The listing builds one solid part. Answer for the finished solid, in the listing's coordinates (mm). A direction names the side the tool comes from. Round coordinates to 2 decimals unless told otherwise and drop trailing zeros. Order: outer loops, then holes, each group sorted by start corner. A loop starts at its lowest first (then second) coordinate and runs counter-clockwise, first axis right, second up. Notation, with made-up numbers: (-9, 62.5) - (34, 62.5) arc R28 cw to (34, 96.5) - close; hole circle Ø7 at (11, 68.5). An arc over 180 degrees is marked (long way). One line per item, written item: value. Start each with the question number.
1. Section A-A, the plane x = 0 is taken. Give the vertices of the cut face in (y, z).
2. A tool of negligible diameter and unlimited length cuts with its end or side. For faces 1 (the flat face through (5.5, -3.12, 3.94)), 2 (the cylindrical face through (2.38, 10.74, 59.04)), 3 (the flat face through (10, -10, 64)), from which of +Z, -Z, +X, -X, +Y, -Y can it reach the whole face along a straight path? Write none if from no direction.
3. Flat-ended cylindrical pins translate along their axes: P1, Ø13, axis at x = 0, y = 0, coming from the +Z side; P2, Ø1.5, axis at y = 12.5, z = 20.5, coming from the +X side; P3, Ø10, axis at x = 15.5, z = 45.5, coming from the +Y side; P4, Ø14, axis at x = 2.5, y = 2.5, coming from the -Z side. Find the tip coordinate at first contact, or state that the pin passes through.
4. Straight lines are drawn through the part: line 1 (Z direction, x = 6, y = 6.5); line 2 (Y direction, x = 0, z = 24); line 3 (Y direction, x = 0, z = 57). For each, find the intervals that lie inside material, in ascending order.
5. For a pull along Y with two mould halves and no side action, classify faces 4 (the flat face through (0, -6.322, 4)), 5 (the flat face through (3, -3, 8)), 6 (the flat face through (0, -8, 0)), 7 (the conical face through (22.72, 7.15, 33.76)) as released by +Y, released by -Y, zero draft, split by the parting line, or undercut.
6. Section B-B, the plane z = 37 is taken. Give the vertices of the cut face in (x, y).
from build123d import *

# Parameters (mm, degrees)
POCKET_DEPTH    = 8
SKETCH003_R     = 3.95
POCKET001_DEPTH = 64.001
SKETCH004_R     = 11
POCKET002_DEPTH = 8
FILLET_R        = 2
FILLET001_R     = 5


with BuildPart() as part:
    # Sketch → Revolution (revolve)
    with BuildSketch(Plane.XZ):
        Polygon((0, 0), (22.5, 0), (25, 64), (0, 64), align=None)
    revolve(axis=Axis((0, 0, 0), (0, 0, 1)))

    # Sketch002 (on Face1 of Revolution) → Pocket (cut)
    with BuildSketch(Plane(origin=(0, 0, 0), x_dir=(1, 0, 0), z_dir=(0, 0, -1))):
        Polygon((7.3, 0), (3.65, 6.321985), (-3.65, 6.321985), (-7.3, 0), (-3.65, -6.321985), (3.65, -6.321985), align=None)
    extrude(amount=-POCKET_DEPTH, mode=Mode.SUBTRACT)

    # Sketch003 (on Face1 of Pocket) → Pocket001 (cut, through all)
    with BuildSketch(Plane(origin=(0, 0, 0), x_dir=(1, 0, 0), z_dir=(0, 0, -1))):
        Circle(SKETCH003_R)
    extrude(amount=-POCKET001_DEPTH, mode=Mode.SUBTRACT)

    # Sketch004 (on Face9 of Pocket001) → Pocket002 (cut)
    with BuildSketch(Plane(origin=(0, 0, 64), x_dir=(-1, 0, 0), z_dir=(0, 0, 1))):
        Circle(SKETCH004_R)
    extrude(amount=-POCKET002_DEPTH, mode=Mode.SUBTRACT)

    # Fillet
    fillet_edges = [part.edges().sort_by_distance(p)[0] for p in [
        (-25, 0, 64),
        (11, 0, 64),
    ]]
    fillet(fillet_edges, radius=FILLET_R)

    # Fillet001
    fillet001_edges = [part.edges().sort_by_distance(p)[0] for p in [
        (-22.5, 0, 0),
    ]]
    fillet(fillet001_edges, radius=FILLET001_R)


solid = part.part
Answer list:
1. outline: (-24.92, 61.92) - (-22.69, 4.8) arc R5 ccw to (-17.69, 0) - (-6.32, 0) - (-6.32, 8) - (-3.95, 8) - (-3.95, 56) - (-11, 56) - (-11, 62) arc R2 ccw to (-13, 64) - (-22.92, 64) arc R2 ccw to start; (3.95, 8) - (6.32, 8) - (6.32, 0) - (17.69, 0) arc R5 ccw to (22.69, 4.8) - (24.92, 61.92) arc R2 ccw to (22.92, 64) - (13, 64) arc R2 ccw to (11, 62) - (11, 56) - (3.95, 56) - close
2. face 1: -Z
2. face 2: +Z
2. face 3: +Z, +X, -X, +Y, -Y
3. P1: stops at z = 56
3. P2: stops at x = 20.12
3. P3: stops at y = 21.9
3. P4: stops at z = 0
4. line 1: z = 0 to 56
4. line 2: y = -23.44 to -3.95, 3.95 to 23.44
4. line 3: y = -24.73 to -11, 11 to 24.73
5. face 4: undercut
5. face 5: undercut
5. face 6: zero draft
5. face 7: split by the parting line
6. outline: circle Ø47.89 at (0, 0); hole circle Ø7.9 at (0, 0)
